Here's how the part is built. I have some questions about the finished solid (model axes, mm). Coordinates: 2 decimals unless noted, no trailing zeros. Loops run counter-clockwise (first coordinate to the right, second up) from the corner with the lowest first, then second, coordinate; pieces in that order, holes last.
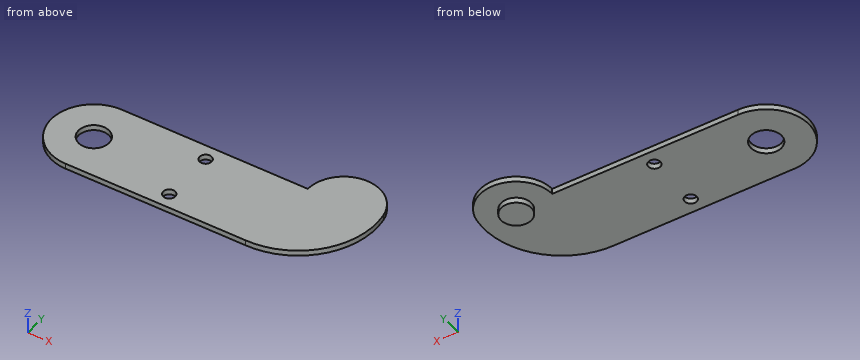
from build123d import *

# Parameters (mm, degrees)
ESBO_O1_R                = 5.05
ESBO_O1_R_2              = 2
RESSALTO_EXTRUS_O1_DEPTH = 1.8
ESBO_O2_R                = 5
RESSALTO_EXTRUS_O2_DEPTH = 1.8


with BuildPart() as part:
    # Esboço1 → Ressalto-extrusão1 (new body)
    with BuildSketch(Plane.XY):
        with BuildLine():
            Line((-12, 0), (-74, 0))
            ThreePointArc((-74, 0), (-88.1, -14.1), (-74, -28.2))
            Line((-74, -28.2), (-14, -28.2))
            ThreePointArc((-14, -28.2), (6.004940765, -19.140656488), (11.826301138, 2.034355278))
            ThreePointArc((11.826301138, 2.034355278), (-1.020878628, 11.956496428), (-12, 0))
        make_face()
        with Locations((-74, -14.1)):
            Circle(ESBO_O1_R, mode=Mode.SUBTRACT)
        with Locations((-42.75, -5)):
            Circle(ESBO_O1_R_2, mode=Mode.SUBTRACT)
        with Locations((-42.75, -23.2)):
            Circle(ESBO_O1_R_2, mode=Mode.SUBTRACT)
    extrude(amount=RESSALTO_EXTRUS_O1_DEPTH)

    # Esboço2 → Ressalto-extrusão2 (add)
    with BuildSketch(Plane.XY):
        Circle(ESBO_O2_R)
    extrude(amount=-RESSALTO_EXTRUS_O2_DEPTH)


solid = part.part
Q1. Suppose I cut it at A-A on z = 1. Write out the boundary of the cut face in (x, y), and give its area (3 significant figures).
Q2. Suppose I cut it at B-B on x = -78. Write out the boundary of the cut face in (y, z), and give its area (3 significant figures).
Q3. Please list where these lines run through material, in increasing order: probe 1 along Y at (x, z) = (-42.75, 1.1); probe 2 along Z at (x, y) = (-61.5, -18); probe 3 along Y at (x, z) = (-74, 0.4).
Q4. Suppose I cut it at D-D on x = 3. Write out the boundary of the cut face in (y, z), and give its area (3 significant figures).
Q5. Suppose I cut it at C-C on y = -14.1. Write out the boundary of the cut face in (x, z), and give its area (3 significant figures).
Q6. Will these pins go through, and if not, where does the flat tip stop? P1, Ø1, axis at y = -14.5, z = -1, coming from the +X side; P2, Ø12, axis at x = -41.5, y = -6, coming from the -Z side; P3, Ø2, axis at x = -36, z = 1, coming from the +Y side; P4, Ø2, axis at x = -34.5, z = 1, coming from the -Y side.
Check values:
1. outline: (-74, -28.2) - (-14, -28.2) arc R25.85 ccw to (11.83, 2.03) arc R12 ccw to (-12, 0) - (-74, 0) arc R14.1 ccw to start; hole circle Ø10.1 at (-74, -14.1); hole circle Ø4 at (-42.75, -23.2); hole circle Ø4 at (-42.75, -5)
1. area: 2,720 mm2
2. outline: (-27.62, 0) - (-17.18, 0) - (-17.18, 1.8) - (-27.62, 1.8) - close; (-11.02, 0) - (-0.58, 0) - (-0.58, 1.8) - (-11.02, 1.8) - close
2. area: 37.6 mm2
3. probe 1: y = -28.2 to -25.2, -21.2 to -7, -3 to 0
3. probe 2: z = 0 to 1.8
3. probe 3: y = -28.2 to -19.15, -9.05 to 0
4. outline: (-22.12, 0) - (-4, 0) - (-4, -1.8) - (4, -1.8) - (4, 0) - (11.62, 0) - (11.62, 1.8) - (-22.12, 1.8) - close
4. area: 75.1 mm2
5. outline: (-88.1, 0) - (-79.05, 0) - (-79.05, 1.8) - (-88.1, 1.8) - close; (-68.95, 0) - (9.38, 0) - (9.38, 1.8) - (-68.95, 1.8) - close
5. area: 157 mm2
6. P1: passes through
6. P2: stops at z = 0
6. P3: stops at y = 0
6. P4: stops at y = -28.2
